Input: part model. Units: mm. Frame: model coordinates. A direction names the side the tool comes from. Give positions to 0.01 mm unless a question says otherwise; leave off trailing zeros. Order: outer loops, then holes, each group sorted by start corner. A loop starts at its lowest first (then second) coordinate and runs counter-clockwise, first axis right, second up. Notation, with made-up numbers: (53, 55.25) - (62, 55.25) arc R10 cw to (62, 71.25) - close; hole circle Ø9 at (-35.5, 79). An arc over 180 degrees is marked (long way). Answer in a Markdown table with one row per item. Add a question column.
1. Access query for faces 4 (the face through (14, 0, 52)), 5 (the face through (16.25, 31, 95)). Directions: +Z, -Z, +X, -X, +Y, -Y. A direction counts if a zero-diameter tool reaches every point of the face in a straight line with its end or side. Return the directions, or none.
2. Section query B-B on y = 29. Return loops of the section in (x, z).
3. Ray query, line 1 (Z direction, x = 12.5, y = 29.5); line 2 (Y direction, x = 18, z = 60); line 3 (X direction, y = 4, z = 58.5). Return the intervals inside material, ascending. Write a range as [from, to].
4. Section query C-C on z = 78. Return loops of the section in (x, y).
5. Mould query, pull axis Y, two halves, no side actions, for faces 1 (the face through (14, 38, 95)), 2 (the face through (24.65, 3.01, 51.79)), 3 (the face through (24.49, 47.15, 51.79)). Classes: released by +Y, released by -Y, zero draft, split by the parting line, or undercut.
6. Contact query for flat-ended pins moving along their axis: pin 1 (5 mm diameter, centred on x = 22.5, z = 55, fed in from +Y); pin 2 (8 mm diameter, centred on x = 24, z = 15, fed in from -Y); pin 3 (12 mm diameter, centred on x = 3, z = 93.5, fed in from -Y). Output: stop coordinate, or through.
7. Section query A-A on z = 96. Return loops of the section in (x, y).
```python
from build123d import *

# Parameters (mm, degrees)
BOSS_EXTRUDE1_DEPTH = 105
FILLET1_R           = 2
CUT_EXTRUDE1_DEPTH  = 20


with BuildPart() as part:
    # Sketch1 → Boss-Extrude1 (new body)
    with BuildSketch(Plane.XY):
        with BuildLine():
            Line((0, 10), (0, 40))
            ThreePointArc((0, 40), (2.928932188, 47.071067812), (10, 50))
            Line((10, 50), (17.5, 50))
            ThreePointArc((17.5, 50), (24.571067812, 47.071067812), (27.5, 40))
            Line((27.5, 40), (27.5, 10))
            ThreePointArc((27.5, 10), (24.571067812, 2.928932188), (17.5, 0))
            Line((17.5, 0), (10, 0))
            ThreePointArc((10, 0), (2.928932188, 2.928932188), (0, 10))
        make_face()
    extrude(amount=BOSS_EXTRUDE1_DEPTH)

    # Fillet1
    fillet1_edges = [part.edges().sort_by_distance(p)[0] for p in [
        (13.75, 50, 0),
        (24.571067812, 47.071067812, 0),
        (27.5, 25, 0),
        (24.571067812, 2.928932188, 0),
        (24.571067812, 47.071067812, 105),
        (13.75, 50, 105),
        (2.928932188, 47.071067812, 105),
        (0, 25, 105),
        (2.928932188, 2.928932188, 105),
        (13.75, 0, 105),
        (24.571067812, 2.928932188, 105),
        (13.75, 0, 0),
        (27.5, 25, 105),
        (2.928932188, 2.928932188, 0),
        (0, 25, 0),
        (2.928932188, 47.071067812, 0),
    ]]
    fillet(fillet1_edges, radius=FILLET1_R)

    # Sketch2 → Cut-Extrude1 (cut)
    with BuildSketch(Plane.XY.offset(105)):
        Polygon((13.75, 38), (11.25, 38), (11.25, 25), (16.25, 25), (16.25, 38), align=None)
    extrude(amount=-CUT_EXTRUDE1_DEPTH, mode=Mode.SUBTRACT)


solid = part.part
```
Answer:
| question | item | result |
|---|---|---|
| 1 | face 4 | +Z, -Z, +X, -X, -Y |
| 1 | face 5 | +Z |
| 2 | outline | (0, 2) arc R2 ccw to (2, 0) - (25.5, 0) arc R2 ccw to (27.5, 2) - (27.5, 103) arc R2 ccw to (25.5, 105) - (16.25, 105) - (16.25, 85) - (11.25, 85) - (11.25, 105) - (2, 105) arc R2 ccw to (0, 103) - close |
| 3 | line 1 | z = [0, 85] |
| 3 | line 2 | y = [0.01, 49.99] |
| 3 | line 3 | x = [2, 25.5] |
| 4 | outline | (0, 10) arc R10 ccw to (10, 0) - (17.5, 0) arc R10 ccw to (27.5, 10) - (27.5, 40) arc R10 ccw to (17.5, 50) - (10, 50) arc R10 ccw to (0, 40) - close |
| 5 | face 1 | undercut |
| 5 | face 2 | released by -Y |
| 5 | face 3 | released by +Y |
| 6 | pin 1 | stops at y = 49.68 |
| 6 | pin 2 | stops at y = 0.32 |
| 6 | pin 3 | stops at y = 0.05 |
| 7 | outline | (0, 10) arc R10 ccw to (10, 0) - (17.5, 0) arc R10 ccw to (27.5, 10) - (27.5, 40) arc R10 ccw to (17.5, 50) - (10, 50) arc R10 ccw to (0, 40) - close; hole (11.25, 25) - (16.25, 25) - (16.25, 38) - (11.25, 38) - close |
